Check sheet for the modelled part. Datum: model origin and axes. Units: mm. A direction names the side the tool comes from. Round coordinates to 2 decimals unless told otherwise and drop trailing zeros. Order: outer loops, then holes, each group sorted by start corner. A loop starts at its lowest first (then second) coordinate and runs counter-clockwise, first axis right, second up.
(1) Mould release check, pull along Y, two halves, no side actions. Record for faces 1 (the flat face through (173, 8, 7.5)), 2 (the flat face through (140.43, 20.12, 0.11)), 3 (the flat face through (188, -23.876, 0)), 4 (the flat face through (188, -25.464, 0)): released by +Y, released by -Y, zero draft, split by the parting line, or undercut.
(2) Sectioned sample at C-C, the plane x = 335. Enter the section's corners in (y, z).
(3) Tool access check on faces 5 (the flat face through (138.92, 19.63, 0.11)), 6 (the flat face through (265.965, 16.457, 0.105)). Record the directions out of +Z, -Z, +X, -X, +Y, -Y that give a thin tool (end or side, any length) a straight path to the whole face; none if there is none.
(4) Sectioned sample at A-A, the plane y = 0. Enter the section's corners in (x, z), and give its area (3 significant figures).
(5) Sectioned sample at D-D, the plane y = 20. Enter the section's corners in (x, z).
(6) Depth check by flat-ended pin: pin 1 (7.5 mm diameter, centred on x = 121, z = 2, fed in from +Y); pin 2 (1 mm diameter, centred on y = -1, z = -4.5, fed in from +X); pin 3 (4 mm diameter, centred on y = -16.5, z = -2.5, fed in from -X). Enter the tip coordinate at first touch or a pass-through.
(7) Thickness scan on probe 1 along Y at (x, z) = (0, 2.5); probe 2 along X at (y, z) = (0, 3.5); probe 3 along Y at (x, z) = (120, -1). Record the ranges inside material, lowest first.
```python
from build123d import *

# Parameters (mm, degrees)
BOSS_EXTRUDE1_DEPTH = 7.5


with BuildPart() as part:
    # Sketch1 → Boss-Extrude1 (new, symmetric)
    with BuildSketch(Plane.XY):
        with BuildLine():
            Line((103.658753776, 7.356207616), (4.476147359, 25.066988991))
            ThreePointArc((4.476147359, 25.066988991), (-25.364178544, 2.246837564), (0, -25.4635))
            Line((0, -25.4635), (381, -25.4635))
            ThreePointArc((381, -25.4635), (406.443730831, 1.003191728), (378.995174246, 25.384454021))
            Line((378.995174246, 25.384454021), (149.724956547, 7.277039279))
            ThreePointArc((149.724956547, 7.277039279), (145.698613571, 8.326503384), (143.18635498, 11.643334619))
            Line((143.18635498, 11.643334619), (137.591783364, 28.84484275))
            ThreePointArc((137.591783364, 28.84484275), (127, 36.5379), (116.408216636, 28.84484275))
            Line((116.408216636, 28.84484275), (110.81364502, 11.643334619))
            ThreePointArc((110.81364502, 11.643334619), (108.038796403, 8.16029732), (103.658753776, 7.356207616))
        make_face()
        with BuildLine():
            Line((0, -23.876), (381, -23.876))
            ThreePointArc((381, -23.876), (404.857463323, 0.940648602), (379.120163383, 23.801882075))
            Line((379.120163383, 23.801882075), (149.849945684, 5.694467333))
            ThreePointArc((149.849945684, 5.694467333), (144.817016963, 7.006297463), (141.676693726, 11.152336508))
            Line((141.676693726, 11.152336508), (136.082122109, 28.353844639))
            ThreePointArc((136.082122109, 28.353844639), (127, 34.9504), (117.917877891, 28.353844639))
            Line((117.917877891, 28.353844639), (112.323306274, 11.152336508))
            ThreePointArc((112.323306274, 11.152336508), (108.854745504, 6.798539884), (103.37969222, 5.793427754))
            Line((103.37969222, 5.793427754), (4.197085803, 23.504209129))
            ThreePointArc((4.197085803, 23.504209129), (-23.782870655, 2.106760409), (0, -23.876))
        make_face(mode=Mode.SUBTRACT)
    extrude(amount=BOSS_EXTRUDE1_DEPTH, both=True)


solid = part.part
```
Derived:
1. face 1: zero draft
1. face 2: released by +Y
1. face 3: undercut
1. face 4: released by -Y
2. outline: (-25.46, -7.5) - (-23.88, -7.5) - (-23.88, 7.5) - (-25.46, 7.5) - close; (20.32, -7.5) - (21.91, -7.5) - (21.91, 7.5) - (20.32, 7.5) - close
3. face 5: +Z, -Z
3. face 6: +Z, -Z, +Y
4. outline: (-25.46, -7.5) - (-23.88, -7.5) - (-23.88, 7.5) - (-25.46, 7.5) - close; (404.88, -7.5) - (406.46, -7.5) - (406.46, 7.5) - (404.88, 7.5) - close
4. area: 47.6 mm2
5. outline: (-15.76, -7.5) - (-13.04, -7.5) - (-13.04, 7.5) - (-15.76, 7.5) - close; (23.82, -7.5) - (32.85, -7.5) - (32.85, 7.5) - (23.82, 7.5) - close; (113.53, -7.5) - (115.2, -7.5) - (115.2, 7.5) - (113.53, 7.5) - close; (138.8, -7.5) - (140.47, -7.5) - (140.47, 7.5) - (138.8, 7.5) - close; (310.82, -7.5) - (330.98, -7.5) - (330.98, 7.5) - (310.82, 7.5) - close; (394.04, -7.5) - (396.76, -7.5) - (396.76, 7.5) - (394.04, 7.5) - close
6. pin 1: stops at y = 36.31
6. pin 2: stops at x = 406.46
6. pin 3: stops at x = -20.93
7. probe 1: y = -25.46 to -23.88, 23.88 to 25.46
7. probe 2: x = -25.46 to -23.88, 404.88 to 406.46
7. probe 3: y = -25.46 to -23.88, 31.9 to 34.06
